For this review, take the finished solid that the model builds, in its own axes (mm). A direction names the side the tool comes from. Round coordinates to 2 decimals unless told otherwise and drop trailing zeros. Order: outer loops, then holes, each group sorted by start corner. A loop starts at its lowest first (then second) coordinate and runs counter-clockwise, first axis right, second up. Notation, with made-up numbers: (6, 20) - (62, 20) arc R12 ccw to (62, 37) - close; hole circle Ø2 at (80, 54). An arc over 180 degrees is marked (long way). Write each question's results on one line, items separated by ' | '. Start each with the question number.
(1) Take a section at B-B, the plane x = -3. Give the boundary of the cut face in (y, z).
(2) For L1, parallel to X at y = 2.1, z = 0; L2, parallel to X at y = 1.3, z = 0; L3, parallel to X at y = 3.95, z = 1.25, list the stretches that pass through material, from the lowest coordinate up. Write a range as from..to.
(3) Draft analysis for pull direction X (two halves, no side actions). For faces 1 (the flat face through (9, 2, 1)), 2 (the cylindrical face through (-0.46, 3.97, 0.56)), 3 (the flat face through (0, 3, 4.5)), state which applies: pulls with the +X half, pulls with the -X half, needs draft (parallel to the pull), parting line crosses it, or undercut.
(4) Take a section at A-A, the plane z = 0. Give the boundary of the cut face in (x, y), plus the area to 3 significant figures.
(5) Take a section at D-D, the plane x = 5.75. Give the boundary of the cut face in (y, z).
(6) For faces 4 (the flat face through (8, 3, 0)), 5 (the flat face through (4, 5, 5)), 6 (the flat face through (0, 1, -4.5)), list the 3-axis set-ups (+Z, -Z, +X, -X, +Y, -Y) from which the entire face can be reached by the end or side of a thin tool; tool diameter is ignored.
(7) Insertion check: pin 1 Ø1 at (x, z) = (5.5, 4.5) entering from +Y; pin 2 Ø4.5 at (x, z) = (2, -2) entering from +Y; pin 3 Ø6 at (x, z) = (2, 0.5) entering from -Y; pin 4 Ø0.9 at (y, z) = (3, 1.5) entering from -X. Each pin has a flat end and moves straight along its axis. Give the tip position at first contact, or say it passes through.
(8) Take a section at C-C, the plane y = 1.5. Give the boundary of the cut face in (x, z).
```python
from build123d import *

# Parameters (mm, degrees)
SKETCH_1_W           = 16
SKETCH_1_H           = 9
EXTRUDE_1_DEPTH      = 2
SKETCH_2_R           = 2.6
EXTRUDE_2_DEPTH      = 4
EXTRUDE_3_DEPTH      = 3
EXTRUDE_3_DEPTH_BACK = 2
SKETCH_4_R           = 1.6
CUT_EXTRUDE_1_DEPTH  = 13.1346611


with BuildPart() as part:
    # 草图1 → 凸台-拉伸1 (new body)
    with BuildSketch(Plane(origin=(0, 0, 0), x_dir=(1, 0, 0), z_dir=(0, 1, 0))):
        Rectangle(SKETCH_1_W, SKETCH_1_H)
    extrude(amount=EXTRUDE_1_DEPTH)

    # 草图2 → 凸台-拉伸2 (add)
    with BuildSketch(Plane(origin=(0, 2, 0), x_dir=(1, 0, 0), z_dir=(0, 1, 0))):
        with Locations(Location((-3, 0, 0), (0, 0, 90))):
            Circle(SKETCH_2_R)
    extrude(amount=EXTRUDE_2_DEPTH)

    # 草图3 → 凸台-拉伸3 (add, two sides: drawn at the far end of the back side and taken through both)
    with BuildSketch(Plane(origin=(0, 2, 0), x_dir=(1, 0, 0), z_dir=(0, 1, 0)).offset(-EXTRUDE_3_DEPTH_BACK)):
        Polygon((-8, -4.5), (-8, -5.5), (9, -5.5), (9, 4.5), (8, 4.5), (8, -4.5), align=None)
    extrude(amount=EXTRUDE_3_DEPTH + EXTRUDE_3_DEPTH_BACK)

    # 草图4 → 切除-拉伸1 (cut, through all)
    with BuildSketch(Plane(origin=(0, 6, 0), x_dir=(1, 0, 0), z_dir=(0, 1, 0))):
        with Locations(Location((-3, 0, 0), (0, 0, 270))):
            Circle(SKETCH_4_R)
    extrude(amount=-CUT_EXTRUDE_1_DEPTH, mode=Mode.SUBTRACT)


solid = part.part
```
Results below:
1) outline: (0, -4.5) - (2, -4.5) - (2, -2.6) - (6, -2.6) - (6, -1.6) - (0, -1.6) - close; (0, 1.6) - (6, 1.6) - (6, 2.6) - (2, 2.6) - (2, 4.5) - (5, 4.5) - (5, 5.5) - (0, 5.5) - close
2) L1: x = -5.6..-4.6, -1.4..-0.4, 8..9 | L2: x = -8..-4.6, -1.4..9 | L3: x = -5.28..-4, -2..-0.72, 8..9
3) face 1: pulls with the +X half | face 2: undercut | face 3: needs draft
4) outline: (-8, 0) - (-4.6, 0) - (-4.6, 6) - (-5.6, 6) - (-5.6, 2) - (-8, 2) - close; (-1.4, 0) - (9, 0) - (9, 5) - (8, 5) - (8, 2) - (-0.4, 2) - (-0.4, 6) - (-1.4, 6) - close | area: 38.6 mm^2
5) outline: (0, -4.5) - (2, -4.5) - (2, 4.5) - (5, 4.5) - (5, 5.5) - (0, 5.5) - close
6) face 4: -Z, +Y | face 5: +Z, +X, +Y | face 6: -Z, +X, -X, +Y, -Y
7) pin 1: stops at y = 5 | pin 2: stops at y = 2 | pin 3: stops at y = 0 | pin 4: stops at x = -5.38
8) outline: (-8, -4.5) - (9, -4.5) - (9, 5.5) - (-8, 5.5) - close; hole circle Ø3.2 at (-3, 0)
